Model file for the job. Use its own axes, mm. A direction names the side the tool comes from. Round coordinates to 2 decimals unless told otherwise and drop trailing zeros. Loops run counter-clockwise (first coordinate to the right, second up) from the corner with the lowest first, then second, coordinate; pieces in that order, holes last. Notation, with made-up numbers: M 81,69.25 L 94,69.25 A20 ccw 94,78.25 Z; hole C 66,11.25 d1. An arc over 180 degrees is marked long. Use a Markdown table: item, result. Add a question column.
Q1. Cut at C-C (y = -21). Give the cut face in (x, z).
Q2. Cut at D-D (x = 18). Give the cut face in (y, z), plus the area to 3 significant figures.
Q3. Mould opens along X. For faces 4 (the face through (15, -5, 5)), 5 (the face through (-25, -10, 2)), 6 (the face through (-19.5, -2.43, 2.46)) say: +X half, -X half, draft (parallel to the pull), parting line (faces both ways), or undercut.
Q4. Probe line 1 (Z direction, x = -16, y = -1); line 2 (Y direction, x = 18, z = 1.1); line 3 (X direction, y = -20.5, z = 0.5). List the from-to ranges inside material, lowest first. Write a range as from..to.
Q5. Pin check, flat tips, straight feed: pin 1 (1 mm diameter, centred on x = 10.5, y = -16, fed in from -Z); pin 2 (3.5 mm diameter, centred on y = -4, z = 7, fed in from +X); pin 3 (4 mm diameter, centred on x = -9.5, z = 1, fed in from -Y); pin 4 (1.5 mm diameter, centred on x = 8.5, z = 5, fed in from -Y). Stop position of each tip, or through.
Q6. Cut at A-A (y = -2.5). Give the cut face in (x, z), plus the area to 3 significant figures.
Q7. Tool access for faces 1 (the face through (17.19, -29.34, 2.46)), 2 (the face through (-1.5, 0, 6)), 3 (the face through (1.5, 0, 6)): list every direction of +Z, -Z, +X, -X, +Y, -Y with a clear straight run to the whole face (end or side of a thin tool).
from build123d import *

# Parameters (mm, degrees)
F0_R        = 1.5
F1_DEPTH    = 5
F2_R        = 5
F3_W        = 3
F3_H        = 21
F4_DEPTH    = 3
F5_R        = 1.5
F6_DEPTH    = 21
F7_T1_DEPTH = 29.0228793414


# Not quite as in the source:
# - a fillet or chamfer that OpenCascade refuses, or shapes differently, is made with other operations: its cross-section is extruded or revolved along the edge and cut away or added


with BuildPart() as f1:
    # F0 (on Top) → F1 (new body)
    with BuildSketch(Plane.XY):
        Polygon((0, -10.5), (25, -10.5), (25, 10.5), (-25, 10.5), (-25, -10.5), align=None)
        with Locations((-18, -2.5)):
            Circle(F0_R, mode=Mode.SUBTRACT)
        with Locations((18, -2.5)):
            Circle(F0_R, mode=Mode.SUBTRACT)
        with BuildLine():
            Line((25, -31), (25, -10.5))
            Line((25, -10.5), (0, -10.5))
            ThreePointArc((0, -10.5), (11.313708499, -15.186291501), (16, -26.5))
            Line((16, -26.5), (16, -31))
            Line((16, -31), (25, -31))
        make_face()
        with BuildLine():
            ThreePointArc((-16, -26.5), (-11.313708499, -15.186291501), (0, -10.5))
            Line((0, -10.5), (-25, -10.5))
            Line((-25, -10.5), (-25, -31))
            Line((-25, -31), (-16, -31))
            Line((-16, -31), (-16, -26.5))
        make_face()
    extrude(amount=F1_DEPTH)

    # F2
    f2_edges = [f1.edges().sort_by_distance(p)[0] for p in [
        (25, -31, 2.5),
        (-25, -31, 2.5),
        (-25, 10.5, 2.5),
        (25, 10.5, 2.5),
    ]]
    fillet(f2_edges, radius=F2_R)

    # F3 (on face) → F4 (join)
    with BuildSketch(Plane.XY.offset(5)):
        Rectangle(F3_W, F3_H)
    extrude(amount=F4_DEPTH)

    # F5 (on face) → F6 (cut, through all)
    with BuildSketch(Plane(origin=(0, 10.5, 0), x_dir=(-1, 0, 0), z_dir=(0, 1, 0))):
        with Locations((0, 8)):
            Circle(F5_R)
    extrude(amount=-F6_DEPTH, mode=Mode.SUBTRACT)

    # F7: fillet of radius 5 on 2 edges, made by hand

    # F7_s2 → F7_t1 (cut)
    with BuildSketch(Plane.XY.offset(-12.0114396707)):
        with BuildLine():
            ThreePointArc((20, -31), (17.1547293043, -29.3007363495), (15.9971008021, -26.1954250064))
            Line((15.9971008021, -26.1954250064), (15.4971914021, -26.204942975))
            ThreePointArc((15.4971914021, -26.204942975), (15.5, -26.5), (15.5, -31))
            Line((15.5, -31), (16, -31.5))
            ThreePointArc((16, -31.5), (18, -31.5), (19.9003805197, -31.4899754679))
            Line((19.9003805197, -31.4899754679), (20, -31))
        make_face()
        with BuildLine():
            ThreePointArc((-20, -31), (-17.1547293043, -29.3007363495), (-15.9971008021, -26.1954250064))
            Line((-15.9971008021, -26.1954250064), (-15.4971914021, -26.204942975))
            ThreePointArc((-15.4971914021, -26.204942975), (-15.5, -26.5), (-15.5, -31))
            Line((-15.5, -31), (-16, -31.5))
            ThreePointArc((-16, -31.5), (-18, -31.5), (-19.9003805197, -31.4899754679))
            Line((-19.9003805197, -31.4899754679), (-20, -31))
        make_face()
    extrude(amount=F7_T1_DEPTH, mode=Mode.SUBTRACT)


solid = f1.part
Checked values:
| question | item | result |
|---|---|---|
| 1 | outline | M -25,0 L -15.02,0 L -15.02,5 L -25,5 Z; M 15.02,0 L 25,0 L 25,5 L 15.02,5 Z |
| 2 | outline | M -30.1,0 L -4,0 L -4,5 L -30.1,5 Z; M -1,0 L 10.5,0 L 10.5,5 L -1,5 Z |
| 2 | area | 188 mm^2 |
| 3 | face 4 | draft |
| 3 | face 5 | -X half |
| 3 | face 6 | undercut |
| 4 | line 1 | z = 0..5 |
| 4 | line 2 | y = -30.1..-4, -1..10.5 |
| 4 | line 3 | x = -25..-14.83, 14.83..25 |
| 5 | pin 1 | passes through |
| 5 | pin 2 | stops at x = 1.5 |
| 5 | pin 3 | stops at y = -15.38 |
| 5 | pin 4 | stops at y = -13.44 |
| 6 | outline | M -25,0 L -19.5,0 L -19.5,5 L -25,5 Z; M -16.5,0 L 16.5,0 L 16.5,5 L 1.5,5 L 1.5,8 A1.5 cw -1.5,8 L -1.5,5 L -16.5,5 Z; M 19.5,0 L 25,0 L 25,5 L 19.5,5 Z |
| 6 | area | 225 mm^2 |
| 7 | face 1 | +Z, -Z, -Y |
| 7 | face 2 | +Z, -X, +Y, -Y |
| 7 | face 3 | +Z, +X, +Y, -Y |
